```python
from build123d import *

# Parameters (mm, degrees)
SKETCH1_R               = 6.5
BOSS_EXTRUDE1_DEPTH     = 36
BOSS_EXTRUDE2_START     = 36
BOSS_EXTRUDE2_DEPTH     = 32
CUT_EXTRUDE1_REACH      = 117.453
SKETCH3_W               = 11
SKETCH3_H               = 15
SKETCH3_H_2             = 8.917737905
SKETCH3_6_R             = 6
CUT_EXTRUDE3_DEPTH      = 11
CUT_EXTRUDE4_DEPTH      = 169.371612809
CUT_EXTRUDE4_DEPTH_BACK = 169.371612809


with BuildPart() as part:
    # Sketch1 → Boss-Extrude1 (new body)
    with BuildSketch(Plane(origin=(0, 0, 0), x_dir=(0, 0, -1), z_dir=(1, 0, 0))):
        Polygon((-12, 90), (-111.955126335, 0), (0, 0), (0, 90), align=None)
        with Locations((-47.636607378, 31)):
            Circle(SKETCH1_R, mode=Mode.SUBTRACT)
        with Locations((-19.871294507, 56)):
            Circle(SKETCH1_R, mode=Mode.SUBTRACT)
    extrude(amount=BOSS_EXTRUDE1_DEPTH)

    # Sketch1<4> → Boss-Extrude2 (add)
    with BuildSketch(Plane(origin=(0, 0, 0), x_dir=(0, 0, -1), z_dir=(1, 0, 0)).offset(BOSS_EXTRUDE2_START)):
        Polygon((-111.955126335, 0), (-94.185326097, 16), (-125, 16), (-125, 0), align=None)
        Polygon((0, 0), (0, 16), (-94.185326097, 16), (-111.955126335, 0), align=None)
    extrude(amount=BOSS_EXTRUDE2_DEPTH)

    # Cut-Extrude1: up to this plane
    cut_extrude1_end = Plane(origin=(36, 0, 0), z_dir=(0, 0, 1))
    # Sketch3 → Cut-Extrude1 (cut, up to the surface)
    with BuildSketch(Plane(origin=(0, 55.670912219, 50.126314512), x_dir=(1, 0, 0), z_dir=(0, 0.7431448254773979, 0.6691306063588541)), mode=Mode.PRIVATE) as cut_extrude1_sk1:
        with Locations((5.5, 43.804016667)):
            Rectangle(SKETCH3_W, SKETCH3_H)
    cut_extrude1_tool1 = split(extrude(cut_extrude1_sk1.sketch, amount=-CUT_EXTRUDE1_REACH, mode=Mode.PRIVATE), bisect_by=cut_extrude1_end, keep=Keep.BOTH, mode=Mode.PRIVATE)
    add(cut_extrude1_tool1.solids().sort_by_distance((5.5, 84.98152, 17.573586))[0], mode=Mode.SUBTRACT)
    # Sketch3 → Cut-Extrude1 (cut, up to the surface)
    with BuildSketch(Plane(origin=(0, 55.670912219, 50.126314512), x_dir=(1, 0, 0), z_dir=(0, 0.7431448254773979, 0.6691306063588541)), mode=Mode.PRIVATE) as cut_extrude1_sk2:
        with Locations((5.5, 55.76288562)):
            Rectangle(SKETCH3_W, SKETCH3_H_2)
    cut_extrude1_tool2 = split(extrude(cut_extrude1_sk2.sketch, amount=-CUT_EXTRUDE1_REACH, mode=Mode.PRIVATE), bisect_by=cut_extrude1_end, keep=Keep.BOTH, mode=Mode.PRIVATE)
    add(cut_extrude1_tool2.solids().sort_by_distance((5.5, 92.983566, 8.686415))[0], mode=Mode.SUBTRACT)

    # Sketch3<6> → Cut-Extrude3 (cut)
    with BuildSketch(Plane(origin=(0, 55.670912219, 50.126314512), x_dir=(1, 0, 0), z_dir=(0, 0.7431448254773979, 0.6691306063588541))):
        with Locations(Location((17, -16.198872821, 0), (0, 0, 270))):
            Circle(SKETCH3_6_R)
    extrude(amount=-CUT_EXTRUDE3_DEPTH, mode=Mode.SUBTRACT)

    # Sketch4 → Cut-Extrude4 (cut, two sides: drawn at the far end of the back side and taken through both)
    with BuildSketch(Plane.XY.offset(125).offset(-CUT_EXTRUDE4_DEPTH_BACK)):
        Polygon((53.698956889, 16), (68, 4), (68, 16), align=None)
    extrude(amount=CUT_EXTRUDE4_DEPTH + CUT_EXTRUDE4_DEPTH_BACK, mode=Mode.SUBTRACT)


solid = part.part
```
Build history of the part. All positions in model axes, mm. A direction names the side the tool comes from. Round coordinates to 2 decimals unless told otherwise and drop trailing zeros. Loops run counter-clockwise (first coordinate to the right, second up) from the corner with the lowest first, then second, coordinate; pieces in that order, holes last.
Item 1: Pin check, flat tips, straight feed: P1, Ø12, axis at x = 7.5, y = 45, coming from the +Z side; P2, Ø17.5, axis at y = 6.5, z = 117, coming from the -X side; P3, Ø6, axis at x = 33, z = 69.5, coming from the +Y side; P4, Ø10.5, axis at y = 31, z = 47.64, coming from the -X side. Stop position of each tip, or through.
Item 2: Saw through at B-B (x = 26). List the corners of the cut face in (y, z).
Item 3: Drill centre lines: line 1 along Y through (x, z) = (40.5, 18.5); line 2 along X through (y, z) = (69, 5.5); line 3 along Y through (x, z) = (28.5, 24). Where is each one in solid material? Low to high.
Item 4: Saw through at C-C (y = 13). List the corners of the cut face in (x, z), then the cut area to 3 significant figures.
Item 5: Saw through at D-D (x = 48). List the corners of the cut face in (y, z).
Item 6: Which spindle directions (+Z, -Z, +X, -X, +Y, -Y) get a long thin tool onto all of the face, cutting with end or side? Do faces 1 (the face through (11, 76, 8)), 2 (the face through (17.084, 36.713, 54.742)), 3 (the face through (25.75, 45.63, 61.28)), 4 (the face through (45, 16, 62)). Say none if no direction does.
Item 7: Saw through at A-A (y = 56). List the corners of the cut face in (x, z).
Item 8: Two-plate mould, pull along X, no slides. Class faces 5 (the face through (17.26, 44.81, 54.08)), 6 (the face through (48, 8, 125)), 7 (the face through (60.749, 10.084, 61.625)): released by +X, released by -X, zero draft, split by the parting line, or undercut.
Worked answers:
1. P1: stops at z = 68.64
1. P2: stops at x = 0
1. P3: stops at y = 40.93
1. P4: passes through
2. outline: (0, 0) - (90, 0) - (90, 12) - (0, 111.96) - close; hole circle Ø13 at (31, 47.64); hole circle Ø13 at (56, 19.87)
3. line 1: y = 0 to 16
3. line 2: x = 11 to 36
3. line 3: y = 0 to 50.98, 61.02 to 79.2
4. outline: (0, 0) - (57.27, 0) - (57.27, 125) - (36, 125) - (36, 97.52) - (0, 97.52) - close
4. area: 6,170 mm2
5. outline: (0, 0) - (16, 0) - (16, 125) - (0, 125) - close
6. face 1: -Z, -X, +Y
6. face 2: none
6. face 3: +Z, -X, +Y
6. face 4: +Z, -Z, +X, +Y
7. outline: (0, 1.57) - (11, 1.57) - (11, 0) - (36, 0) - (36, 13.37) - (0, 13.37) - close; (0, 26.37) - (36, 26.37) - (36, 49.76) - (0, 49.76) - close
8. face 5: undercut
8. face 6: zero draft
8. face 7: released by +X
